Could you check a few things on this drawing? It's one solid part, dimensions in mm from its lowest x, y, z. Give positions to 0.01 mm unless a question says otherwise; leave off trailing zeros. Loops run counter-clockwise (first coordinate to the right, second up) from the corner with the lowest first, then second, coordinate; pieces in that order, holes last. Notation, with made-up numbers: M -38.5,75 L 1.5,75 A29 ccw 1.5,114 Z; hole C 74,22 d9. An arc over 180 degrees is marked long. Answer in a Markdown table with one row per item. Add a question column.
1. I'm going to push flat-ended pins straight in: pin 1 Ø1.5 at (x, y) = (200, 20) entering from -Z (1 decimal); pin 2 Ø1 at (y, z) = (21, 197.5) entering from +X (1 decimal); pin 3 Ø10 at (x, z) = (131.5, 132) entering from -Y. Where does each tip first touch, or does it pass through?
2. I need wall thicknesses on line 1 along X through (y, z) = (11.25, 30) (1 decimal); line 2 along Y through (x, z) = (270.5, 179); line 3 along Z through (x, y) = (102, 26) (1 decimal). Which ranges of each line are inside material? Lowest first, please. Write a range as from..to.
3. If we section it at C-C on x = 60.5: List the corners of the cut face in (y, z) for me (1 decimal), then the cut area to 3 significant figures.
4. If we section it at B-B on z = 80.5: List the corners of the cut face in (x, y) for me (1 decimal).
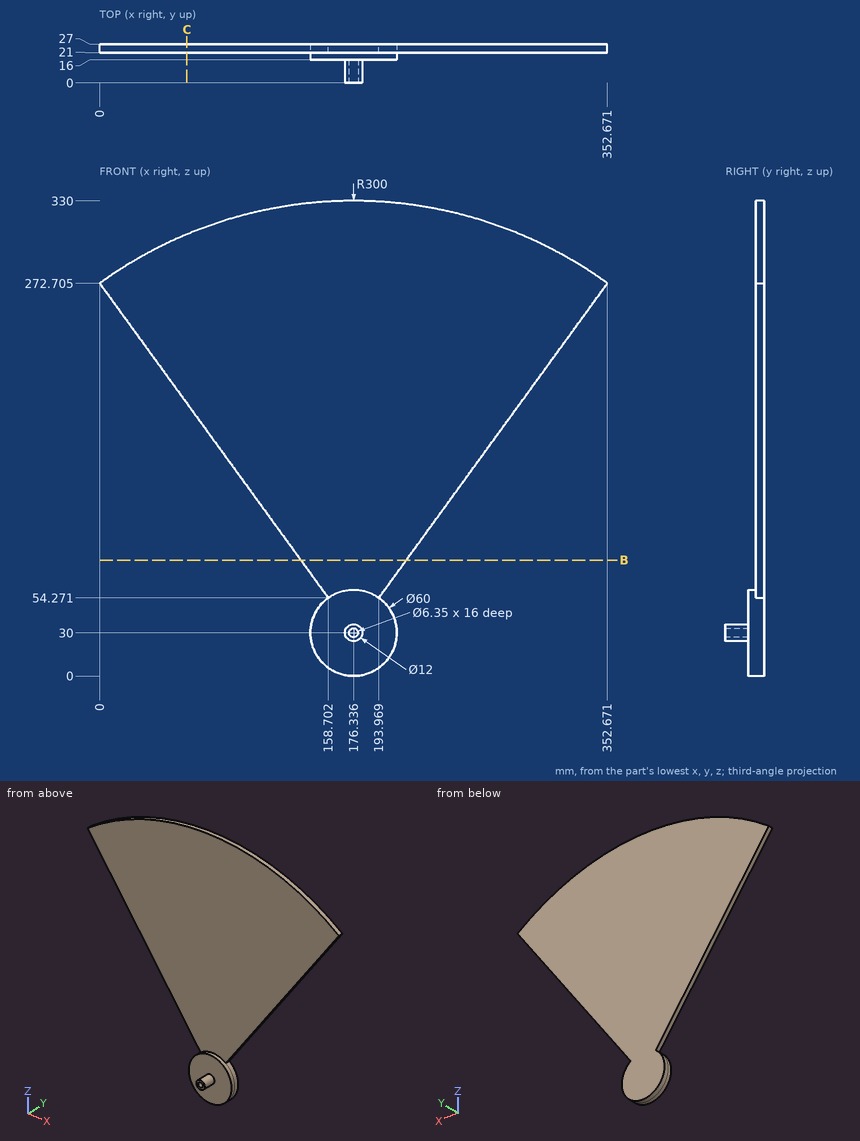
Results:
| question | item | result |
|---|---|---|
| 1 | pin 1 | z = 10.6 |
| 1 | pin 2 | x = 298.4 |
| 1 | pin 3 | y = 21 |
| 2 | line 1 | 170.3..173.2, 179.5..182.3 |
| 2 | line 2 | 21..27 |
| 2 | line 3 | 132.3..320.6 |
| 3 | outline | M 21,189.4 L 27,189.4 L 27,306.7 L 21,306.7 Z |
| 3 | area | 704 mm2 |
| 4 | outline | M 139.6,21 L 213,21 L 213,27 L 139.6,27 Z |
